Here's how the part is built. I have some questions about the finished solid (model axes, mm). Give positions to 0.01 mm unless a question says otherwise; leave off trailing zeros. Loops run counter-clockwise (first coordinate to the right, second up) from the corner with the lowest first, then second, coordinate; pieces in that order, holes last.
Q1. If we section it at C-C (y = 21): Please give me the cut outline in (x, z), plus the area to 3 significant figures.
Q2. If we section it at D-D (z = 13): Please give me the cut outline in (x, y), plus the area to 3 significant figures.
Q3. If we section it at B-B (z = -20): Please give me the cut outline in (x, y), plus the area to 3 significant figures.
Q4. Will these pins go through, and if not, where does the flat tip stop? P1, Ø3.5, axis at y = 17.75, z = -30.74, coming from the -X side; P2, Ø0.6, axis at x = 1, y = -32.5, coming from the -Z side; P3, Ø1, axis at x = 1, y = -31.5, coming from the +Z side; P4, Ø1, axis at x = 1.5, z = -14, coming from the -Y side.
Q5. I need wall thicknesses on line 1 (Y direction, x = 1.5, z = 25); line 2 (Z direction, x = 1.6, y = 33); line 3 (Z direction, x = 0.75, y = 9). Which ranges of each line are inside material? Lowest first, please.
Q6. If we section it at A-A (y = -17.75): Please give me the cut outline in (x, z), plus the area to 3 significant figures.
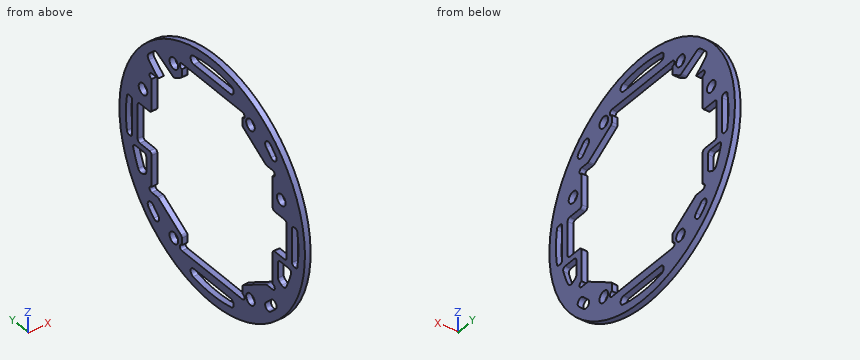
from build123d import *

# Parameters (mm, degrees)
SKETCH_1_R          = 42.95
SKETCH_1_R_2        = 2
EXTRUDE_1_DEPTH     = 2
SKETCH_5_R          = 1
SKETCH_5_R_2        = 2
SKETCH_5_W          = 14
SKETCH_5_H          = 6.5
CUT_EXTRUDE_2_DEPTH = 61.773390559
CUT_EXTRUDE_3_DEPTH = 61.773390559
FILLET_1_R          = 1


with BuildPart() as part:
    # 草图1 → 凸台-拉伸1 (new body)
    with BuildSketch(Plane(origin=(0, 0, 0), x_dir=(0, 0, -1), z_dir=(1, 0, 0))):
        Circle(SKETCH_1_R)
        with Locations((-30.743901834, 17.75)):
            Circle(SKETCH_1_R_2, mode=Mode.SUBTRACT)
        with Locations(Location((-30.743901834, -17.75, 0), (0, 0, 180))):
            Circle(SKETCH_1_R_2, mode=Mode.SUBTRACT)
        with Locations((30.743901834, -17.75)):
            Circle(SKETCH_1_R_2, mode=Mode.SUBTRACT)
        with Locations(Location((30.743901834, 17.75, 0), (0, 0, 180))):
            Circle(SKETCH_1_R_2, mode=Mode.SUBTRACT)
        Polygon((-21, 28), (21, 28), (21, 25), (28, 14), (33, 14), (33, -14), (28, -14), (21, -25), (21, -28), (-21, -28), (-21, -25), (-28, -14), (-33, -14), (-33, 14), (-28, 14), (-21, 25), align=None, mode=Mode.SUBTRACT)
    extrude(amount=EXTRUDE_1_DEPTH)

    # 草图5 → 切除-拉伸2 (cut, through all)
    with BuildSketch(Plane(origin=(2, 0, 0), x_dir=(0, 0, -1), z_dir=(1, 0, 0))):
        with Locations((32, 14)):
            Circle(SKETCH_5_R)
        with Locations((20, 28)):
            Circle(SKETCH_5_R)
        with Locations((-20, 28)):
            Circle(SKETCH_5_R)
        with Locations((-32, 14)):
            Circle(SKETCH_5_R)
        with Locations((-32, -14)):
            Circle(SKETCH_5_R)
        with Locations((-20, -28)):
            Circle(SKETCH_5_R)
        with Locations((20, -28)):
            Circle(SKETCH_5_R)
        with Locations((32, -14)):
            Circle(SKETCH_5_R)
        with Locations((-13, 32)):
            Circle(SKETCH_5_R_2)
        with Locations(Location((-13, -32, 0), (0, 0, 180))):
            Circle(SKETCH_5_R_2)
        with BuildLine():
            Line((-36, 8.49426277), (-36, -8.49426277))
            ThreePointArc((-36, -8.49426277), (-37.333279159, -9.984968697), (-38.962938882, -8.82563843))
            ThreePointArc((-38.962938882, -8.82563843), (-39.95, 0), (-38.962938882, 8.82563843))
            ThreePointArc((-38.962938882, 8.82563843), (-37.333279159, 9.984968697), (-36, 8.49426277))
        make_face()
        with Locations((0, 31.25)):
            Rectangle(SKETCH_5_W, SKETCH_5_H)
        with BuildLine():
            Line((-7, 39.331952659), (-7, 37))
            Line((-7, 37), (7, 37))
            Line((7, 37), (7, 39.331952659))
            ThreePointArc((7, 39.331952659), (0, 39.95), (-7, 39.331952659))
        make_face()
        with BuildLine():
            Line((9, 30.5), (9, 36.867363616))
            ThreePointArc((9, 36.867363616), (12.719592996, 35.754922095), (16.306065038, 34.268276043))
            ThreePointArc((16.306065038, 34.268276043), (17.093879667, 33.359276514), (16.960594644, 32.163798729))
            Line((16.960594644, 32.163798729), (16, 30.5))
            Line((16, 30.5), (9, 30.5))
        make_face()
        with BuildLine():
            Line((36, 8.49426277), (36, -8.49426277))
            ThreePointArc((36, -8.49426277), (37.333279159, -9.984968697), (38.962938882, -8.82563843))
            ThreePointArc((38.962938882, -8.82563843), (39.95, 0), (38.962938882, 8.82563843))
            ThreePointArc((38.962938882, 8.82563843), (37.333279159, 9.984968697), (36, 8.49426277))
        make_face()
        with Locations((0, -31.25)):
            Rectangle(SKETCH_5_W, SKETCH_5_H)
        with BuildLine():
            Line((16, -30.5), (9, -30.5))
            Line((9, -30.5), (9, -36.867363616))
            ThreePointArc((9, -36.867363616), (12.719592996, -35.754922095), (16.306065038, -34.268276043))
            ThreePointArc((16.306065038, -34.268276043), (17.093879667, -33.359276514), (16.960594644, -32.163798729))
            Line((16.960594644, -32.163798729), (16, -30.5))
        make_face()
        with BuildLine():
            Line((7, -39.331952659), (7, -37))
            Line((7, -37), (-7, -37))
            Line((-7, -37), (-7, -39.331952659))
            ThreePointArc((-7, -39.331952659), (0, -39.95), (7, -39.331952659))
        make_face()
        with BuildLine():
            ThreePointArc((-26.996751137, 29.44788495), (-28.248915908, 28.248915908), (-29.44788495, 26.996751137))
            ThreePointArc((-29.44788495, 26.996751137), (-29.357386268, 24.91275018), (-27.273385311, 25.003248863))
            ThreePointArc((-27.273385311, 25.003248863), (-26.162950904, 26.162950904), (-25.003248863, 27.273385311))
            ThreePointArc((-25.003248863, 27.273385311), (-24.91275018, 29.357386268), (-26.996751137, 29.44788495))
        make_face()
        with BuildLine():
            ThreePointArc((26.996751137, 29.44788495), (28.248915908, 28.248915908), (29.44788495, 26.996751137))
            ThreePointArc((29.44788495, 26.996751137), (29.357386268, 24.91275018), (27.273385311, 25.003248863))
            ThreePointArc((27.273385311, 25.003248863), (26.162950904, 26.162950904), (25.003248863, 27.273385311))
            ThreePointArc((25.003248863, 27.273385311), (24.91275018, 29.357386268), (26.996751137, 29.44788495))
        make_face()
        with BuildLine():
            ThreePointArc((26.996751137, -29.44788495), (28.248915908, -28.248915908), (29.44788495, -26.996751137))
            ThreePointArc((29.44788495, -26.996751137), (29.357386268, -24.91275018), (27.273385311, -25.003248863))
            ThreePointArc((27.273385311, -25.003248863), (26.162950904, -26.162950904), (25.003248863, -27.273385311))
            ThreePointArc((25.003248863, -27.273385311), (24.91275018, -29.357386268), (26.996751137, -29.44788495))
        make_face()
        with BuildLine():
            ThreePointArc((-26.996751137, -29.44788495), (-28.248915908, -28.248915908), (-29.44788495, -26.996751137))
            ThreePointArc((-29.44788495, -26.996751137), (-29.357386268, -24.91275018), (-27.273385311, -25.003248863))
            ThreePointArc((-27.273385311, -25.003248863), (-26.162950904, -26.162950904), (-25.003248863, -27.273385311))
            ThreePointArc((-25.003248863, -27.273385311), (-24.91275018, -29.357386268), (-26.996751137, -29.44788495))
        make_face()
    extrude(amount=-CUT_EXTRUDE_2_DEPTH, mode=Mode.SUBTRACT)

    # 草图6 → 切除-拉伸3 (cut, through all)
    with BuildSketch(Plane(origin=(2, 0, 0), x_dir=(0, 0, -1), z_dir=(1, 0, 0))):
        Polygon((-29.668633505, 25.318263062), (-25.674311866, 17.654652782), (-21, 25), (-24.902514308, 29.346104641), align=None)
    extrude(amount=-CUT_EXTRUDE_3_DEPTH, mode=Mode.SUBTRACT)

    # 圆角1
    fillet_1_edges = [part.edges().sort_by_distance(p)[0] for p in [
        (1, -36.867363616, -9),
        (1, -30.5, -9),
        (1, -30.5, -16),
        (1, -39.331952659, -7),
        (1, -39.331952659, 7),
        (1, -37, 7),
        (1, -37, -7),
        (1, -14, 28),
        (1, -25, 21),
        (1, 30.5, -16),
        (1, -25, -21),
        (1, 30.5, -9),
        (1, 36.867363616, -9),
        (1, -14, -28),
        (1, 34.5, -7),
        (1, 28, -7),
        (1, 28, 7),
        (1, 34.5, 7),
        (1, 14, -28),
        (1, 25, -21),
        (1, 39.331952659, 7),
        (1, 39.331952659, -7),
        (1, 37, -7),
        (1, 37, 7),
        (1, 14, 28),
        (1, -34.5, 7),
        (1, -28, 7),
        (1, -28, -7),
        (1, -34.5, -7),
        (1, 17.654652782, 25.674311866),
    ]]
    fillet(fillet_1_edges, radius=FILLET_1_R)


solid = part.part
Check sheet entries:
1. outline: (0, -37.47) - (2, -37.47) - (2, -23.55) - (0, -23.55) - close; (0, 27.42) - (2, 27.42) - (2, 37.47) - (0, 37.47) - close
1. area: 47.9 mm2
2. outline: (0, -40.94) - (2, -40.94) - (2, -34) - (0, -34) - close; (0, -30) - (2, -30) - (2, -28) - (0, -28) - close; (0, 28) - (2, 28) - (2, 30) - (0, 30) - close; (0, 34) - (2, 34) - (2, 40.94) - (0, 40.94) - close
2. area: 35.7 mm2
3. outline: (0, -38.01) - (2, -38.01) - (2, -29) - (0, -29) - close; (0, 29) - (2, 29) - (2, 38.01) - (0, 38.01) - close
3. area: 36.0 mm2
4. P1: passes through
4. P2: stops at z = -28.42
4. P3: stops at z = 29.73
4. P4: stops at y = -40.77
5. line 1: y = -34.92 to -29.44, -27.28 to -18.71, 29.44 to 34.92
5. line 2: z = -27.49 to -17.16, -9 to -7, 7 to 11.27, 14.73 to 27.49
5. line 3: z = -42 to -38.91, -36.09 to -33, 33 to 36.09, 38.91 to 42
6. outline: (0, -39.11) - (2, -39.11) - (2, -32.74) - (0, -32.74) - close; (0, -28.74) - (2, -28.74) - (2, -25.61) - (0, -25.61) - close; (0, 25.61) - (2, 25.61) - (2, 28.74) - (0, 28.74) - close; (0, 32.74) - (2, 32.74) - (2, 39.11) - (0, 39.11) - close
6. area: 38.0 mm2
